Design review of the part built by this model. Coordinates are the model's own, in mm. Round coordinates to 2 decimals unless told otherwise and drop trailing zeros. Loops run counter-clockwise (first coordinate to the right, second up) from the corner with the lowest first, then second, coordinate; pieces in that order, holes last. Notation, with made-up numbers: (12, 71.25) -> (23, 71.25) arc R6 cw to (23, 76.25) -> close; hole circle Ø5 at (40, 62.25). An arc over 180 degrees is marked (long way). Answer as CSV lines item,"result". Start each with the question number.
```python
from build123d import *

# Parameters (mm, degrees)
SKETCH1_W           = 12
SKETCH1_H           = 400
BOSS_EXTRUDE1_DEPTH = 8
CUT_EXTRUDE1_DEPTH  = 401
SKETCH3_R           = 3
CUT_EXTRUDE2_DEPTH  = 4.5
SKETCH4_R           = 1.75
CUT_EXTRUDE3_DEPTH  = 4.5
LPATTERN1_COUNT     = 16
LPATTERN1_PITCH     = 25


with BuildPart() as part:
    # Sketch1 → Boss-Extrude1 (new body)
    with BuildSketch(Plane.XY):
        with Locations((0, 200)):
            Rectangle(SKETCH1_W, SKETCH1_H)
    extrude(amount=BOSS_EXTRUDE1_DEPTH)

    # Sketch2 → Cut-Extrude1 (cut, through all)
    with BuildSketch(Plane(origin=(0, 400, 0), x_dir=(1, 0, 0), z_dir=(0, 1, 0))):
        with BuildLine():
            Line((-5.5, 0), (-6, -0.5))
            Line((-6, -0.5), (-6, -3.5))
            ThreePointArc((-6, -3.5), (-5.867156742, -4.117156742), (-5.492156742, -4.625))
            ThreePointArc((-5.492156742, -4.625), (-5.322875656, -5), (-5.492156742, -5.375))
            ThreePointArc((-5.492156742, -5.375), (-5.90312152, -7.030330086), (-4.5, -8))
            Line((-4.5, -8), (-7.760322007, -8))
            Line((-7.760322007, -8), (-7.760322007, 0))
            Line((-7.760322007, 0), (-5.5, 0))
        make_face()
        with BuildLine():
            Line((6, -0.5), (6, -3.5))
            ThreePointArc((6, -3.5), (5.867156742, -4.117156742), (5.492156742, -4.625))
            ThreePointArc((5.492156742, -4.625), (5.322875656, -5), (5.492156742, -5.375))
            ThreePointArc((5.492156742, -5.375), (5.90312152, -7.030330086), (4.5, -8))
            Line((4.5, -8), (7.760322007, -8))
            Line((7.760322007, -8), (7.760322007, 0))
            Line((7.760322007, 0), (5.5, 0))
            Line((5.5, 0), (6, -0.5))
        make_face()
    extrude(amount=-CUT_EXTRUDE1_DEPTH, mode=Mode.SUBTRACT)

    # Sketch3 → Cut-Extrude2 (cut)
    with BuildSketch(Plane.XY.offset(8)):
        with Locations((0, 390)):
            Circle(SKETCH3_R)
    cut_extrude2 = extrude(amount=-CUT_EXTRUDE2_DEPTH, mode=Mode.SUBTRACT)

    # Sketch4 → Cut-Extrude3 (cut, through all)
    with BuildSketch(Plane.XY.offset(3.5)):
        with Locations((0, 390)):
            Circle(SKETCH4_R)
    cut_extrude3 = extrude(amount=-CUT_EXTRUDE3_DEPTH, mode=Mode.SUBTRACT)

    # LPattern1: Cut-Extrude2, Cut-Extrude3 ×16
    with Locations(*[(0, -i * LPATTERN1_PITCH, 0) for i in range(1, LPATTERN1_COUNT)]):
        add(cut_extrude2, mode=Mode.SUBTRACT)
        add(cut_extrude3, mode=Mode.SUBTRACT)


solid = part.part
```
Q1. For pin 1 Ø6.5 at (x, y) = (-1, 65) entering from +Z; pin 2 Ø1.8 at (x, y) = (0.5, 389) entering from +Z, all flat-tipped, find the tip position at first contact; note any pin that passes through.
Q2. To check wall thickness, follow probe 1 along X at (y, z) = (390, 1.75); probe 2 along X at (y, z) = (40, 4.5); probe 3 along X at (y, z) = (205, 7.5). State the ranges of each line that lie inside material, in increasing order. Write a range as from..to.
Q3. Add section A-A, the plane y = 358. Give the boundary of the cut face in (x, z) (3 decimals), and give its area (3 significant figures).
Worked answers:
1,pin 1,"stops at z = 8"
1,pin 2,"stops at z = 3.5"
2,probe 1,"x = -6..-1.75, 1.75..6"
2,probe 2,"x = -5.62..-3, 3..5.62"
2,probe 3,"x = -5.62..5.62"
3,outline,"(-6, 0.5) -> (-5.5, 0) -> (5.5, 0) -> (6, 0.5) -> (6, 3.5) arc R1.5 ccw to (5.492, 4.625) arc R0.5 cw to (5.492, 5.375) arc R1.5 ccw to (4.5, 8) -> (-4.5, 8) arc R1.5 ccw to (-5.492, 5.375) arc R0.5 cw to (-5.492, 4.625) arc R1.5 ccw to (-6, 3.5) -> close"
3,area,"93.1 mm^2"
